For this review, take the finished solid that the model builds, in its own axes (mm). Face numbers are marked on the shaded views. A direction names the side the tool comes from. Coordinates: 2 decimals unless noted, no trailing zeros. Loops run counter-clockwise (first coordinate to the right, second up) from the corner with the lowest first, then second, coordinate; pieces in that order, holes last.
1. To check wall thickness, follow probe 1 along X at (y, z) = (-16, 1.5); probe 2 along X at (y, z) = (-4.5, 1); probe 3 along X at (y, z) = (6, 1). State the ranges of each line that lie inside material, in increasing order.
2. Take a section at A-A, the plane y = -4. State the section outline as (x, z) points, then the cut area to 3 significant figures.
3. Clearance check with flat-ended pins moving along their axes: P1, Ø3.5, axis at x = 0, z = 4, coming from the +Y side; P2, Ø1.3, axis at y = -14, z = 4.5, coming from the +X side; P3, Ø1.5, axis at x = -21.5, z = 3.5, coming from the +Y side. State where each tip first meets the part, or that it passes through.
4. Take a section at D-D, the plane x = -19. State the section outline as (y, z) points, then the cut area to 3 significant figures.
5. Take a section at B-B, the plane x = 21. State the section outline as (y, z) points, then the cut area to 3 significant figures.
6. Take a section at C-C, the plane z = 7. State the section outline as (x, y) points, then the cut area to 4 significant figures.
7. Machinability: for the marked faces 1 and 2, which of the approach directions +Z, -Z, +X, -X, +Y, -Y give a long, thin tool a straight path to every point of the face, cutting with its end or side? Answer none if there is none.
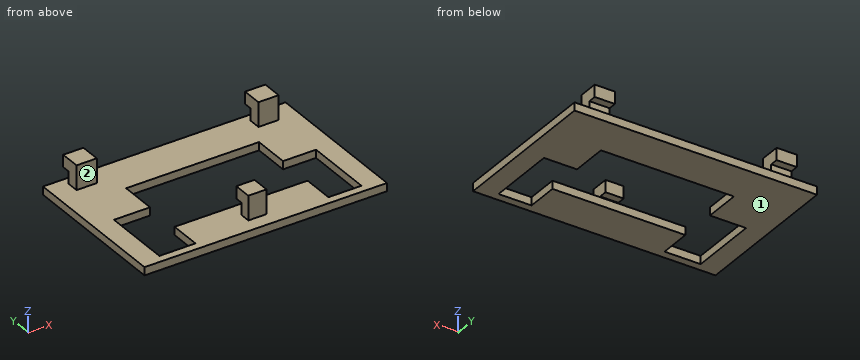
```python
from build123d import *

# Parameters (mm, degrees)
F0_W     = 60
F0_H     = 38
F0_W_2   = 4.5
F0_H_2   = 2.5
F0_W_3   = 5
F0_H_3   = 3
F1_DEPTH = 2
F2_DEPTH = 8
F3_W     = 5
F3_H     = 3
F4_DEPTH = 2
F5_W     = 5
F5_H     = 3
F6_DEPTH = 2
F7_DEPTH = 8
F8_W     = 4.5
F8_H     = 3
F9_DEPTH = 2


# Not quite as in the source:
# - a feature names something its author has since deleted; it is built from what else it names


with BuildPart() as f1:
    # F0 (on Top) → F1 (new body)
    with BuildSketch(Plane.XY):
        Rectangle(F0_W, F0_H)
        with Locations((0.25, -14.25)):
            Rectangle(F0_W_2, F0_H_2, mode=Mode.SUBTRACT)
        Polygon((-16.0694369525, 0), (-16.0694369525, 8.9702934623), (16.8300806135, 8.9702934623), (16.8300806135, 0), (25, 0), (25, -17), (16.8300806135, -17), (16.8300806135, -9.1921526343), (-16.0694369525, -9.1921526343), (-16.0694369525, -17), (-25, -17), (-25, 0), align=None, mode=Mode.SUBTRACT)
        with Locations((-22.5, 15.5)):
            Rectangle(F0_W_3, F0_H_3, mode=Mode.SUBTRACT)
        with Locations((22.5, 15.5)):
            Rectangle(F0_W_3, F0_H_3, mode=Mode.SUBTRACT)
    extrude(amount=F1_DEPTH)

    # F0 (on Top) → F2 (join)
    with BuildSketch(Plane.XY):
        with Locations((22.5, 15.5)):
            Rectangle(F0_W_3, F0_H_3)
        with Locations((-22.5, 15.5)):
            Rectangle(F0_W_3, F0_H_3)
    extrude(amount=F2_DEPTH)

    # F3 (on face) → F4 (join)
    with BuildSketch(Plane(origin=(0, 17, 0), x_dir=(-1, 0, 0), z_dir=(0, 1, 0))):
        with Locations((22.5, 6.5)):
            Rectangle(F3_W, F3_H)
    extrude(amount=F4_DEPTH)

    # F5 (on face) → F6 (join)
    with BuildSketch(Plane(origin=(0, 17, 0), x_dir=(-1, 0, 0), z_dir=(0, 1, 0))):
        with Locations((-22.5, 6.5)):
            Rectangle(F5_W, F5_H)
    extrude(amount=F6_DEPTH)

    # F0 (on Top) → F7 (join)
    with BuildSketch(Plane.XY):
        with Locations((0.25, -14.25)):
            Rectangle(F0_W_2, F0_H_2)
    extrude(amount=F7_DEPTH)

    # F8 (on face) → F9 (join)
    with BuildSketch(Plane(origin=(0, -13, 0), x_dir=(-1, 0, 0), z_dir=(0, 1, 0))):
        with Locations((-0.25, 6.5)):
            Rectangle(F8_W, F8_H)
    extrude(amount=F9_DEPTH)


solid = f1.part
```
Results list:
1. probe 1: x = -30 to -25, -16.07 to 16.83, 25 to 30
1. probe 2: x = -30 to -25, 25 to 30
1. probe 3: x = -30 to -16.07, 16.83 to 30
2. outline: (-30, 0) - (-25, 0) - (-25, 2) - (-30, 2) - close; (25, 0) - (30, 0) - (30, 2) - (25, 2) - close
2. area: 20.0 mm2
3. P1: stops at y = -11
3. P2: stops at x = 2.5
3. P3: stops at y = 17
4. outline: (-19, 0) - (-17, 0) - (-17, 2) - (-19, 2) - close; (0, 0) - (19, 0) - (19, 2) - (0, 2) - close
4. area: 42.0 mm2
5. outline: (-19, 0) - (-17, 0) - (-17, 2) - (-19, 2) - close; (0, 0) - (19, 0) - (19, 2) - (17, 2) - (17, 5) - (19, 5) - (19, 8) - (14, 8) - (14, 2) - (0, 2) - close
5. area: 66.0 mm2
6. outline: (-25, 14) - (-20, 14) - (-20, 19) - (-25, 19) - close; (-2, -15.5) - (2.5, -15.5) - (2.5, -11) - (-2, -11) - close; (20, 14) - (25, 14) - (25, 19) - (20, 19) - close
6. area: 70.25 mm2
7. face 1: -Z, +X, -X, +Y, -Y
7. face 2: +Z, +X, -X, -Y
